from build123d import *

# Parameters (mm, degrees)
SKETCH1_R           = 1.7
SKETCH1_R_2         = 1.5875
BOSS_EXTRUDE1_DEPTH = 2
SKETCH2_W           = 56.4
SKETCH2_H           = 2
BOSS_EXTRUDE2_DEPTH = 56.4
SKETCH3_R           = 19.05
SKETCH3_R_2         = 1.5
CUT_EXTRUDE1_DEPTH  = 94.696531419


with BuildPart() as part:
    # Sketch1 → Boss-Extrude1 (new body)
    with BuildSketch(Plane(origin=(0, 0, 0), x_dir=(1, 0, 0), z_dir=(0, 1, 0))):
        Polygon((0, 43.275), (50.8, 43.275), (50.8, -9.525), (38.1, -9.525), (38.1, 0), (0, 0), align=None)
        with Locations(Location((44.45, 36.5125, 0), (0, 0, 270))):
            Circle(SKETCH1_R, mode=Mode.SUBTRACT)
        with Locations(Location((44.45, -4.7625, 0), (0, 0, 270))):
            Circle(SKETCH1_R, mode=Mode.SUBTRACT)
        with Locations(Location((9.525, 15.875, 0), (0, 0, 270))):
            Circle(SKETCH1_R_2, mode=Mode.SUBTRACT)
        with Locations(Location((41.275, 15.875, 0), (0, 0, 270))):
            Circle(SKETCH1_R_2, mode=Mode.SUBTRACT)
    extrude(amount=BOSS_EXTRUDE1_DEPTH)

    # Sketch2 → Boss-Extrude2 (add)
    with BuildSketch(Plane(origin=(0, 2, 0), x_dir=(1, 0, 0), z_dir=(0, 1, 0))):
        with Locations((22.6, 42.275)):
            Rectangle(SKETCH2_W, SKETCH2_H)
    extrude(amount=BOSS_EXTRUDE2_DEPTH)

    # Sketch3 → Cut-Extrude1 (cut, through all)
    with BuildSketch(Plane(origin=(0, 0, -43.275), x_dir=(-1, 0, 0), z_dir=(0, 0, -1))):
        with Locations((-22.6, 30.2)):
            Circle(SKETCH3_R)
        with Locations((0.95, 53.75)):
            Circle(SKETCH3_R_2)
        with Locations((0.95, 6.65)):
            Circle(SKETCH3_R_2)
        with Locations((-46.15, 6.65)):
            Circle(SKETCH3_R_2)
        with Locations((-46.15, 53.75)):
            Circle(SKETCH3_R_2)
    extrude(amount=-CUT_EXTRUDE1_DEPTH, mode=Mode.SUBTRACT)


solid = part.part
Can you work these out from the model? Positions are in its coordinate system, mm. A direction names the side the tool comes from. Coordinates: 2 decimals unless noted, no trailing zeros. Order: outer loops, then holes, each group sorted by start corner. A loop starts at its lowest first (then second) coordinate and runs counter-clockwise, first axis right, second up. Notation, with made-up numbers: M 20,-16 L 37,-16 A26 ccw 37,9 Z; hole C 71.5,71.25 d3. An arc over 180 degrees is marked long. Write item = value, one per line.
(1) For faces 1 (the face through (38.1, 1, 5)), 2 (the face through (4.43, 35.92, -42.29)), 3 (the face through (-3, 2, -42)), 4 (the face through (22, 11, -41.275)), which set-ups out of +Z, -Z, +X, -X, +Y, -Y let a thin tool reach every point of the face, with its end or its side?
Results are:
face_1 = +Z, -X, +Y, -Y
face_2 = +Z, -Z
face_3 = +Z, -Z, -X, -Y
face_4 = +Z, +X, -X, +Y
(2) Suppose I cut it at D-D on x = 22.6. Please give me the cut outline in (y, z) (3 decimals).
Results are:
outline = M 0,-43.275 L 11.15,-43.275 L 11.15,-41.275 L 2,-41.275 L 2,0 L 0,0 Z; M 49.25,-43.275 L 58.4,-43.275 L 58.4,-41.275 L 49.25,-41.275 Z
(3) I need wall thicknesses on line 1 along Y through (x, z) = (22.6, -42.85); line 2 along Y through (x, z) = (33, -2); line 3 along Z through (x, y) = (21.5, 54.5) (3 decimals). Which ranges of each line are inside material? Lowest first, please. Write a range as [from, to].
Results are:
line_1 = [0, 11.15], [49.25, 58.4]
line_2 = [0, 2]
line_3 = [-43.275, -41.275]
(4) Suppose I cut it at A-A on x = -0.95. Please give me the cut outline in (y, z) (3 decimals), plus the area to 3 significant figures.
Results are:
outline = M 2,-43.275 L 5.15,-43.275 L 5.15,-41.275 L 2,-41.275 Z; M 8.15,-43.275 L 52.25,-43.275 L 52.25,-41.275 L 8.15,-41.275 Z; M 55.25,-43.275 L 58.4,-43.275 L 58.4,-41.275 L 55.25,-41.275 Z
area = 101 mm2
(5) For pin 1 Ø4 at (x, z) = (44.45, 4.76) entering from +Y; pin 2 Ø2 at (x, z) = (-2.5, -42.5) entering from -Y; pin 3 Ø2 at (x, y) = (15, 10.5) entering from +Z (3 decimals), each with a flat end and sliding along its axis, tell me the tip position at first contact or that it passes through.
Results are:
pin_1 = 2
pin_2 = 2
pin_3 = -41.275
(6) Suppose I cut it at B-B on y = 30.2. Please give me the cut outline in (x, z) (3 decimals), plus the area to 3 significant figures.
Results are:
outline = M -5.6,-43.275 L 3.55,-43.275 L 3.55,-41.275 L -5.6,-41.275 Z; M 41.65,-43.275 L 50.8,-43.275 L 50.8,-41.275 L 41.65,-41.275 Z
area = 36.6 mm2
(7) Suppose I cut it at C-C on y = 6.65. Please give me the cut outline in (x, z) (3 decimals).
Results are:
outline = M -5.6,-43.275 L -2.45,-43.275 L -2.45,-41.275 L -5.6,-41.275 Z; M 0.55,-43.275 L 44.65,-43.275 L 44.65,-41.275 L 0.55,-41.275 Z; M 47.65,-43.275 L 50.8,-43.275 L 50.8,-41.275 L 47.65,-41.275 Z
(8) If we mould it in two halves opening along Z, with no side actions, what happens to faces 5 (the face through (39.725, 0.986, -16.219)), 6 (the face through (9.7, 15.8, -43.275)), 7 (the face through (47.26, 7.66, -42.29))? For each: pulls with the +Z half, pulls with the -Z half, needs draft (parallel to the pull), parting line crosses it, or undercut.
Results are:
face_5 = undercut
face_6 = pulls with the -Z half
face_7 = needs draft
